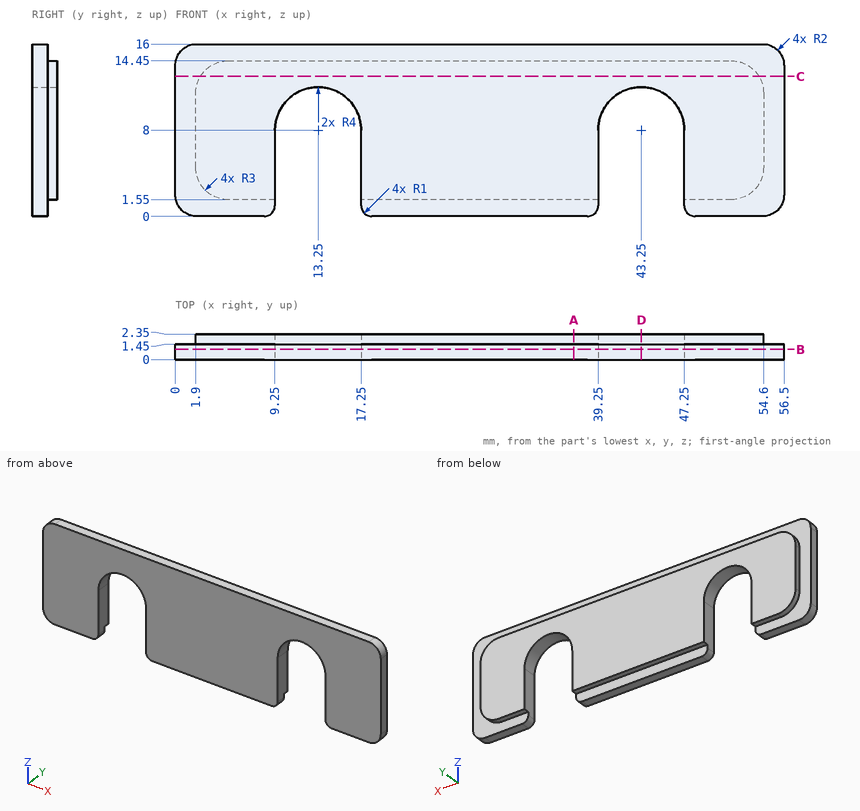
Source: three-view drawing plus pictorial views. Frame: mm from the lowest corner of the part. Give positions to 0.01 mm unless a question says otherwise; leave off trailing zeros. Loops run counter-clockwise (first coordinate to the right, second up) from the corner with the lowest first, then second, coordinate; pieces in that order, holes last. Notation, with made-up numbers: (65, -34) -> (69, -34) arc R20 cw to (69, 4) -> close; hole circle Ø5 at (51, 74). An arc over 180 degrees is marked (long way). Put each result on its own line as item: value. Start each with the question number.
1) Cut plane B-B (y = 0.95). Return loops of the section in (x, z).
2) Cut plane C-C (z = 13). Return loops of the section in (x, y), then the cut area to 3 significant figures.
3) Contact query for flat-ended pins moving along their axis: P1, Ø0.5, axis at x = 8, y = 2, coming from the -Z side; P2, Ø0.5, axis at y = 2, z = 7, coming from the -X side; P3, Ø0.5, axis at x = 26, z = 1, coming from the +Y side. Output: stop coordinate, or through.
4) Cut plane D-D (x = 43.25). Return loops of the section in (y, z), then the cut area to 4 significant figures.
5) Material intervals for probe 1 along X at (y, z) = (0.55, 4.5); probe 2 along X at (y, z) = (2.1, 7.75); probe 3 along Z at (x, y) = (51.5, 1.7), sorted ascending.
6) Cut plane A-A (x = 37). Return loops of the section in (y, z).
Results are:
1. outline: (0, 2) arc R2 ccw to (2, 0) -> (8.25, 0) arc R1 ccw to (9.25, 1) -> (9.25, 8) arc R4 cw to (17.25, 8) -> (17.25, 1) arc R1 ccw to (18.25, 0) -> (38.25, 0) arc R1 ccw to (39.25, 1) -> (39.25, 8) arc R4 cw to (47.25, 8) -> (47.25, 1) arc R1 ccw to (48.25, 0) -> (54.5, 0) arc R2 ccw to (56.5, 2) -> (56.5, 14) arc R2 ccw to (54.5, 16) -> (2, 16) arc R2 ccw to (0, 14) -> close
2. outline: (0, 0) -> (56.5, 0) -> (56.5, 1.45) -> (54.17, 1.45) -> (54.17, 2.35) -> (2.33, 2.35) -> (2.33, 1.45) -> (0, 1.45) -> close
2. area: 129 mm2
3. P1: stops at z = 1.55
3. P2: stops at x = 1.9
3. P3: stops at y = 1.45
4. outline: (0, 12) -> (2.35, 12) -> (2.35, 14.45) -> (1.45, 14.45) -> (1.45, 16) -> (0, 16) -> close
4. area: 8.005 mm2
5. probe 1: x = 0 to 9.25, 17.25 to 39.25, 47.25 to 56.5
5. probe 2: x = 1.9 to 9.25, 17.25 to 39.25, 47.25 to 54.6
5. probe 3: z = 1.55 to 14.45
6. outline: (0, 0) -> (1.45, 0) -> (1.45, 1.55) -> (2.35, 1.55) -> (2.35, 14.45) -> (1.45, 14.45) -> (1.45, 16) -> (0, 16) -> close
